Autodesk Inventor part; units mm, degrees
ref_plane "YZ Plane" through (0, 0, 0) normal (1, 0, 0) x (0, 1, 0)
ref_plane "XZ Plane" through (0, 0, 0) normal (0, 1, 0) x (-1, 0, 0)
ref_plane "XY Plane" through (0, 0, 0) normal (0, 0, 1) x (1, 0, 0)
sketch "Эскиз1" plane through (0, 0, 0) normal (0, 1, 0) x (-1, 0, 0)
  circle A0 centre (0, 0) radius 8.75
  circle A1 centre (0, 0) radius 1.5
  circle A2 centre (0, 0) radius 3
  circle A3 centre (0, 0) radius 7.25
  point P0 (-0.5625, 2.9468)
  point P1 (-0.6797, 7.2181)
  point P2 (0.6797, 7.2181)
  point P3 (0.5625, 2.9468)
  dimension "d1" = 3
  dimension "d2" = 6
  dimension "d24" = 17.5
  dimension "d41" = 1.5
extrude "Выдавливание1" add sketch "Эскиз1" along normal blind 8 contours A0
extrude "Выдавливание7" add sketch "Эскиз1" along normal blind 6 contours A2
extrude "Выдавливание8" add sketch "Эскиз1" along normal blind 1.75 contours A3
properties part number "Колесо заднее"
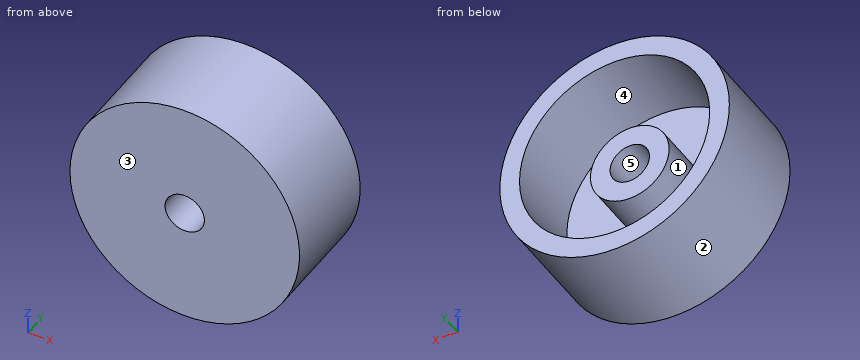
Could you check a few things on this model? Use its own coordinates, in mm. Face numbers are marked on the shaded views. A direction names the side the tool comes from. Give positions to 0.01 mm unless a question says otherwise; leave off trailing zeros. Order: outer loops, then holes, each group sorted by start corner. A loop starts at its lowest first (then second) coordinate and runs counter-clockwise, first axis right, second up.
Q1. I'm going to push flat-ended pins straight in: P1, Ø2, axis at y = 6.5, z = 6.5, coming from the +X side; P2, Ø3, axis at x = 0, z = -0.5, coming from the +Y side; P3, Ø1, axis at y = 4, z = -3.5, coming from the -X side. Where does each tip first touch, or does it pass through?
Q2. Suppose I cut it at A-A, the plane y = 4.5. Write out the boundary of the cut face in (x, z).
Q3. We'd pull the mould along X, two halves only. Please class the marked faces 1, 2 and 3: +X half, -X half, draft (parallel to the pull), parting line (faces both ways), or undercut.
Q4. Suppose I cut it at B-B, the plane z = 0. Write out the boundary of the cut face in (x, y), and give its area (3 significant figures).
Q5. Suppose I cut it at C-C, the plane x = 0. Write out the boundary of the cut face in (y, z), and give its area (3 significant figures).
Q6. Suppose I cut it at D-D, the plane x = -5.25. Write out the boundary of the cut face in (y, z), and give its area (3 significant figures).
Q7. For the marked faces 4 and 5, which set-ups out of +Z, -Z, +X, -X, +Y, -Y let a thin tool reach every point of the face, with its end or its side?
Q8. If I drill on line 1 along Z through (x, y) = (0, 2.95); line 2 along X through (y, z) = (5.25, 1.75); line 3 along Z through (x, y) = (0, 6.25), over which ranges is the centre line in solid material (lowest first)?
Solution:
1. P1: stops at x = 6.81
1. P2: stops at y = 6
1. P3: stops at x = -8.22
2. outline: circle Ø17.5 at (0, 0); circle Ø6 at (0, 0); hole circle Ø14.5 at (0, 0); hole circle Ø3 at (0, 0)
3. face 1: undercut
3. face 2: parting line
3. face 3: draft
4. outline: (-8.75, 0) - (-1.5, 0) - (-1.5, 6) - (-3, 6) - (-3, 1.75) - (-7.25, 1.75) - (-7.25, 8) - (-8.75, 8) - close; (1.5, 0) - (8.75, 0) - (8.75, 8) - (7.25, 8) - (7.25, 1.75) - (3, 1.75) - (3, 6) - (1.5, 6) - close
4. area: 56.9 mm2
5. outline: (0, -8.75) - (8, -8.75) - (8, -7.25) - (1.75, -7.25) - (1.75, -3) - (6, -3) - (6, -1.5) - (0, -1.5) - close; (0, 1.5) - (6, 1.5) - (6, 3) - (1.75, 3) - (1.75, 7.25) - (8, 7.25) - (8, 8.75) - (0, 8.75) - close
5. area: 56.9 mm2
6. outline: (0, -7) - (8, -7) - (8, -5) - (1.75, -5) - (1.75, 5) - (8, 5) - (8, 7) - (0, 7) - close
6. area: 49.5 mm2
7. face 4: +Y
7. face 5: +Y, -Y
8. line 1: z = -8.75 to -7.25, -3 to -1.5, 1.5 to 3, 7.25 to 8.75
8. line 2: x = -8.57 to -7.04, -2.44 to 2.44, 7.04 to 8.57
8. line 3: z = -8.75 to -7.25, 7.25 to 8.75
